Input: part model. Units: mm. Frame: model coordinates. A direction names the side the tool comes from. Coordinates: 2 decimals unless noted, no trailing zeros. Order: outer loops, then holes, each group sorted by start corner. A loop starts at its lowest first (then second) coordinate and runs counter-clockwise, first axis right, second up. Notation, with made-up numbers: (-21, -29.5) - (9, -29.5) arc R19 cw to (9, 7.5) - close; hole circle Ø1 at (80, -28). An arc over 180 degrees is marked (long way). Use a Markdown table: item, result. Add a question column.
Autodesk Fusion 360 part; units mm, degrees
sketch "Sketch1" plane through (0, 0, 0) normal (0, 1, 0) x (1, 0, 0)
  line L0 (-39.9507, -29.6666) -> (-39.6666, -29.6666)
  line L1 (-39.9507, -29.6666) -> (-39.9507, 40)
  line L2 (-39.9507, 40) -> (-50, 40)
  line L3 (-50, 40) -> (-50, -29.6666)
  line L4 (-39.9507, -29.6666) -> (40, -29.6666)
  line L5 (40, -29.6666) -> (40, -40)
  line L6 (40, -40) -> (-39.9507, -40)
  line L7 (-50, -40) -> (-50, -29.6666)
  line L8 (-50, -40) -> (-39.9507, -40)
extrude "Extrude1" add sketch "Sketch1" along normal blind 100
sketch "Sketch2" plane through (-39.9507, 0, 0) normal (1, 0, 0) x (0, 1, 0)
  line L0 (0, 29.6666) -> (0, -40)
  line L1 (0, -40) -> (100, -40)
  line L2 (100, -40) -> (100, 29.6666)
  line L3 (100, 29.6666) -> (0, 29.6666)
  circle A0 centre (10, 20) radius 6
  circle A1 centre (90, 20) radius 6
  circle A2 centre (10, -30) radius 6
  circle A3 centre (90, -30) radius 6
  dimension "d3" = 12
  dimension "d6" = 80
  dimension "d7" = -50
extrude "Extrude2" cut sketch "Sketch2" against normal up to surface (10.0493 mm away) contours A0 | A1 | A2 | A3
1) Pull-direction query (Z, two-part tool) for faces 1 (the flat face through (-4, 49, 40)), 2 (the cylindrical face through (-44.905, 8.699, -35.857)), 3 (the flat face through (-25, 100, 32)), 4 (the cylindrical face through (-45, 84, 20)); classes: pulls with the +Z half, pulls with the -Z half, needs draft (parallel to the pull), parting line crosses it, or undercut.
2) Material intervals for L1, parallel to Z at x = -43, y = 90; L2, parallel to X at y = 24, z = -8; L3, parallel to Z at x = 25, y = 25.5, sorted ascending.
3) Cut plane A-A (z = 20). Return the cut outline in (x, y), and give its area (3 significant figures).
4) Reachability of faces 5 (the flat face through (-39.951, 49, -5)), 6 (the cylindrical face through (-44.91, 85.24, -33.65)) from +Z, -Z, +X, -X, +Y, -Y: full face, straight path, thin tool, end or side. Return the list, or none.
5) Cut plane B-B (y = 10). Return the cut outline in (x, z), and give its area (3 significant figures).
6) Cut plane D-D (y = 41). Return the cut outline in (x, z), and give its area (3 significant figures).
7) Contact query for flat-ended pins moving along their axis: P1, Ø2, axis at y = 50.5, z = -12, coming from the +X side; P2, Ø5, axis at x = -29.5, y = 45.5, coming from the -Z side. Output: stop coordinate, or through.
8) Cut plane C-C (x = -25). Return the cut outline in (y, z).
Computed:
| question | item | result |
|---|---|---|
| 1 | face 1 | pulls with the +Z half |
| 1 | face 2 | undercut |
| 1 | face 3 | needs draft |
| 1 | face 4 | undercut |
| 2 | L1 | z = -40 to -36, -24 to 14, 26 to 40 |
| 2 | L2 | x = -50 to -39.95 |
| 2 | L3 | z = 29.67 to 40 |
| 3 | outline | (-50, 0) - (-39.95, 0) - (-39.95, 4) - (-50, 4) - close; (-50, 16) - (-39.95, 16) - (-39.95, 84) - (-50, 84) - close; (-50, 96) - (-39.95, 96) - (-39.95, 100) - (-50, 100) - close |
| 3 | area | 764 mm2 |
| 4 | face 5 | -Z, +X, +Y, -Y |
| 4 | face 6 | +X, -X |
| 5 | outline | (-50, -40) - (-39.95, -40) - (-39.95, -36) - (-50, -36) - close; (-50, -24) - (-39.95, -24) - (-39.95, 14) - (-50, 14) - close; (-50, 26) - (-39.95, 26) - (-39.95, 29.67) - (40, 29.67) - (40, 40) - (-50, 40) - close |
| 5 | area | 1,390 mm2 |
| 6 | outline | (-50, -40) - (-39.95, -40) - (-39.95, 29.67) - (40, 29.67) - (40, 40) - (-50, 40) - close |
| 6 | area | 1,630 mm2 |
| 7 | P1 | stops at x = -39.95 |
| 7 | P2 | stops at z = 29.67 |
| 8 | outline | (0, 29.67) - (100, 29.67) - (100, 40) - (0, 40) - close |
